Answer from the drawing. Dimensions are ordinates in mm from the lowest x, y and z of the part. A direction names the side the tool comes from. Round coordinates to 2 decimals unless told otherwise and drop trailing zeros. Loops run counter-clockwise (first coordinate to the right, second up) from the corner with the lowest first, then second, coordinate; pieces in that order, holes last. Notation, with made-up numbers: M 10.25,-39 L 45.25,-39 A20 ccw 45.25,-4 Z; hole C 13.25,27.5 d9. An arc over 180 degrees is marked long. Answer as CSV lines item,"result".
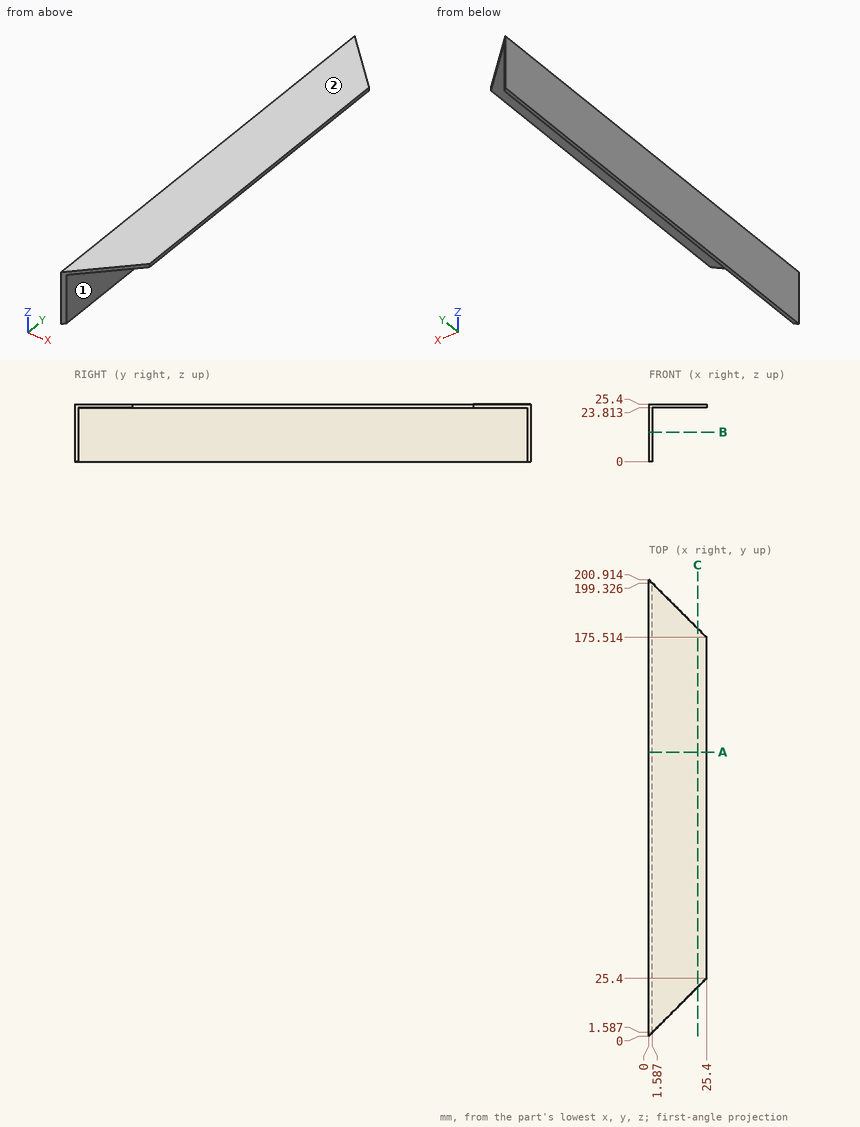
1) This flat-tipped pin is pushed along its axis until it touches: P1, Ø2, axis at y = 59, z = 4.5, coming from the +X side. Where does it stop, or does it pass through?
Evaluation:
P1,"stops at x = 1.59"
2) Find section A-A, the plane y = 125. Give the vertices of the cut face in (x, z).
Evaluation:
outline,"M 0,0 L 1.59,0 L 1.59,23.81 L 25.4,23.81 L 25.4,25.4 L 0,25.4 Z"
3) Find section C-C, the plane x = 21.5. Give the vertices of the cut face in (y, z) (1 decimal).
Evaluation:
outline,"M 21.5,23.8 L 179.4,23.8 L 179.4,25.4 L 21.5,25.4 Z"
4) Find section B-B, the plane z = 13. Give the vertices of the cut face in (x, y) (1 decimal).
Evaluation:
outline,"M 0,0 L 1.6,1.6 L 1.6,199.3 L 0,200.9 Z"
5) Straight lines are drawn through the part: line 1 (Z direction, x = 11.25, y = 26); line 2 (X direction, y = 132, z = 14.25); line 3 (Y direction, x = 20, z = 24.25) (1 decimal). For each, find the intervals that lie inside material, in ascending order.
Evaluation:
line 1,"z = 23.81 to 25.4"
line 2,"x = 0 to 1.59"
line 3,"y = 20 to 180.9"
6) A tool of negligible diameter and unlimited length cuts with its end or side. For the marked faces 1 and 2, from which of +Z, -Z, +X, -X, +Y, -Y can it reach the whole face along a straight path? Write none if from no direction.
Evaluation:
face 1,"-Z, +X, +Y, -Y"
face 2,"+Z, +X, -X, +Y, -Y"
